Geometry check sheet. Reference: the model listing, model coordinates, mm. A direction names the side the tool comes from. Give positions to 0.01 mm unless a question says otherwise; leave off trailing zeros. Write each loop counter-clockwise with the first axis right and the second up, starting at its lowest first coordinate (ties: lowest second). Pieces come first, ordered by that corner, then holes.
(1) Cross-section at C-C (y = -12). Record the boundary of the cut face in (x, z) (3 decimals).
(2) Depth check by flat-ended pin: P1, Ø0.5, axis at y = -8, z = 4, coming from the -X side; P2, Ø1, axis at x = 12, y = -24, coming from the +Z side. Enter the tip coordinate at first touch or a pass-through.
(3) Cross-section at A-A (y = -6.75). Record the boundary of the cut face in (x, z).
(4) Cross-section at D-D (x = 19.75). Record the boundary of the cut face in (y, z).
(5) Tool access check on faces 3 (the flat face through (3, -5, 4)), 4 (the flat face through (11.875, -27, 1)), 5 (the flat face through (14, -9.4, 1)). Record the directions out of +Z, -Z, +X, -X, +Y, -Y that give a thin tool (end or side, any length) a straight path to the whole face; none if there is none.
(6) Cross-section at B-B (x = 13). Count the separate pieces of the cut face and the enclosed holes in it, and give its area (3 significant figures).
(7) Thickness scan on line 1 along Y through (x, z) = (12.25, 1.4); line 2 along Y through (x, z) = (16.25, 3.15); line 3 along X through (y, z) = (-14.75, 3). Record the ranges inside material, lowest first.
(8) Mould release check, pull along X, two halves, no side actions. Record for faces 1 (the flat face through (3, -8, 4)), 2 (the flat face through (22, -14, 2)): +X half, -X half, draft (parallel to the pull), parting line (faces both ways), or undercut.
Autodesk Inventor part; units mm, degrees
ref_plane "YZ Plane" through (0, 0, 0) normal (1, 0, 0) x (0, 1, 0)
ref_plane "XZ Plane" through (0, 0, 0) normal (0, 1, 0) x (-1, 0, 0)
ref_plane "XY Plane" through (0, 0, 0) normal (0, 0, 1) x (1, 0, 0)
sketch "Sketch1" plane through (0, 0, 0) normal (0, 0, 1) x (1, 0, 0)
  line L0 (0, 0) -> (22, 0)
  line L1 (22, 0) -> (22, -29)
  line L2 (22, -29) -> (0, -29)
  line L3 (0, -29) -> (0, 0)
  line L4 (3, -5.35) -> (19, -5.35)
  line L5 (19, -5.35) -> (19, -7.65)
  line L6 (19, -7.65) -> (3, -7.65)
  line L7 (3, -7.65) -> (3, -5.35)
  line L8 (3, -13.35) -> (19, -13.35)
  line L9 (19, -13.35) -> (19, -15.65)
  line L10 (19, -15.65) -> (3, -15.65)
  line L11 (3, -15.65) -> (3, -13.35)
  line L12 (3, -21.35) -> (19, -21.35)
  line L13 (19, -21.35) -> (19, -23.65)
  line L14 (19, -23.65) -> (3, -23.65)
  line L15 (3, -23.65) -> (3, -21.35)
  line L16 (19, -5.35) -> (19, -13.35) construction
  line L17 (19, -13.35) -> (19, -21.35) construction
  line L18 (22, -14.5) -> (0, -14.5) construction
  line L19 (11, 0) -> (11, -29) construction
  point P0 (19, -14.5)
  point P1 (11, -5.35)
  dimension "d0" = 22
  dimension "d1" = 29
  dimension "d2" = 2.3
  dimension "d3" = 8
  dimension "d4" = 16
extrude "Body with light pipe slots" add sketch "Sketch1" along normal blind 4.5
sketch "Sketch2" plane through (0, 0, 4.5) normal (0, 0, 1) x (1, 0, 0)
  line L0 (0, -29) -> (22, -29) construction
  line L1 (22, -29) -> (22, 0) construction
  line L2 (22, 0) -> (0, 0) construction
  line L3 (0, 0) -> (0, -29) construction
  line L4 (3, -21.35) -> (19, -21.35) construction
  line L5 (19, -21.35) -> (19, -23.65) construction
  line L6 (19, -23.65) -> (3, -23.65) construction
  line L7 (3, -23.65) -> (3, -21.35) construction
  line L8 (3, -13.35) -> (19, -13.35) construction
  line L9 (19, -13.35) -> (19, -15.65) construction
  line L10 (19, -15.65) -> (3, -15.65) construction
  line L11 (3, -15.65) -> (3, -13.35) construction
  line L12 (3, -5.35) -> (19, -5.35) construction
  line L13 (19, -5.35) -> (19, -7.65) construction
  line L14 (19, -7.65) -> (3, -7.65) construction
  line L15 (3, -7.65) -> (3, -5.35) construction
  line L16 (1, -5.35) -> (21, -5.35)
  line L17 (21, -5.35) -> (21, -7.65)
  line L18 (21, -7.65) -> (1, -7.65)
  line L19 (1, -7.65) -> (1, -5.35)
  line L20 (1, -13.35) -> (21, -13.35)
  line L21 (21, -13.35) -> (21, -15.65)
  line L22 (21, -15.65) -> (1, -15.65)
  line L23 (1, -15.65) -> (1, -13.35)
  line L24 (1, -21.35) -> (21, -21.35)
  line L25 (21, -21.35) -> (21, -23.65)
  line L26 (21, -23.65) -> (1, -23.65)
  line L27 (1, -23.65) -> (1, -21.35)
  dimension "d7" = 2
  dimension "d8" = 2
extrude "Light pipe wing cuts" cut sketch "Sketch2" against normal blind 4
sketch "Sketch3" plane through (0, 0, 4.5) normal (0, 0, 1) x (1, 0, 0)
  line L0 (1, -21.35) -> (21, -21.35) construction
  line L1 (21, -21.35) -> (21, -23.65) construction
  line L2 (21, -23.65) -> (1, -23.65) construction
  line L3 (1, -23.65) -> (1, -21.35) construction
  line L4 (1, -13.35) -> (21, -13.35) construction
  line L5 (21, -13.35) -> (21, -15.65) construction
  line L6 (21, -15.65) -> (1, -15.65) construction
  line L7 (1, -15.65) -> (1, -13.35) construction
  line L8 (1, -5.35) -> (21, -5.35) construction
  line L9 (21, -5.35) -> (21, -7.65) construction
  line L10 (21, -7.65) -> (1, -7.65) construction
  line L11 (1, -7.65) -> (1, -5.35) construction
  line L12 (0, -29) -> (22, -29) construction
  line L13 (22, -29) -> (22, 0) construction
  line L14 (22, 0) -> (0, 0) construction
  line L15 (0, 0) -> (0, -29) construction
  line L16 (3, -5.35) -> (3, -7.65) construction
  line L17 (19, -7.65) -> (19, -5.35) construction
  line L18 (19, -15.65) -> (19, -13.35) construction
  line L19 (19, -23.65) -> (19, -21.35) construction
  line L20 (3, -21.35) -> (3, -23.65) construction
  line L21 (3, -13.35) -> (3, -15.65) construction
  line L22 (3, -4.35) -> (19, -4.35)
  line L23 (19, -4.35) -> (19, -8.65)
  line L24 (19, -8.65) -> (3, -8.65)
  line L25 (3, -8.65) -> (3, -4.35)
  line L26 (3, -12.35) -> (19, -12.35)
  line L27 (19, -12.35) -> (19, -16.65)
  line L28 (19, -16.65) -> (3, -16.65)
  line L29 (3, -16.65) -> (3, -12.35)
  line L30 (3, -20.2545) -> (19, -20.2545)
  line L31 (19, -20.2545) -> (19, -24.5545)
  line L32 (19, -24.5545) -> (3, -24.5545)
  line L33 (3, -24.5545) -> (3, -20.2545)
  dimension "d11" = 1
  dimension "d12" = 1
  dimension "d13" = 1.0956
  dimension "d14" = 1
extrude "SMD clearance cuts" cut sketch "Sketch3" against normal blind 1
sketch "Sketch4" plane through (0, 0, 0) normal (0, 0, -1) x (-1, 0, 0)
  line L0 (-22, 0) -> (0, 0) construction
  line L1 (-11, 0) -> (-11, -29) construction
  line L2 (0, -29) -> (-22, -29) construction
  line L3 (-11.875, 0) -> (-10.125, 0)
  line L4 (-10.125, -29) -> (-11.875, -29)
  line L5 (-3, -5.35) -> (-19, -5.35)
  line L6 (-19, -23.65) -> (-3, -23.65)
  line L7 (-6.75, -23.65) -> (-6.75, -25.4)
  line L8 (-15.25, -25.4) -> (-15.25, -23.65)
  line L9 (-19, -15.65) -> (-3, -15.65)
  line L10 (-6.75, -15.65) -> (-6.75, -17.4)
  line L11 (-15.25, -17.4) -> (-15.25, -15.65)
  line L12 (-3, -7.65) -> (-19, -7.65)
  line L13 (-6.75, -7.65) -> (-6.75, -9.4)
  line L14 (-15.25, -9.4) -> (-15.25, -7.65)
  line L15 (-11.875, -7.65) -> (-11.875, 0)
  line L16 (-10.125, 0) -> (-10.125, -7.65)
  line L17 (-6.75, -9.4) -> (-10.125, -9.4)
  line L18 (-11.875, -9.4) -> (-15.25, -9.4)
  line L19 (-11.875, -15.65) -> (-11.875, -9.4)
  line L20 (-10.125, -9.4) -> (-10.125, -15.65)
  line L21 (-15.25, -15.65) -> (-11.875, -15.65)
  line L22 (-10.125, -15.65) -> (-6.75, -15.65)
  line L23 (-6.75, -17.4) -> (-10.125, -17.4)
  line L24 (-11.875, -17.4) -> (-15.25, -17.4)
  line L25 (-15.25, -23.65) -> (-11.875, -23.65)
  line L26 (-10.125, -23.65) -> (-6.75, -23.65)
  line L27 (-6.75, -25.4) -> (-10.125, -25.4)
  line L28 (-11.875, -25.4) -> (-15.25, -25.4)
  line L29 (-11.875, -29) -> (-11.875, -25.4)
  line L30 (-11.875, -23.65) -> (-11.875, -17.4)
  line L31 (-10.125, -17.4) -> (-10.125, -23.65)
  line L32 (-10.125, -25.4) -> (-10.125, -29)
  line L33 (-15.25, -7.65) -> (-11.875, -7.65)
  line L34 (-10.125, -7.65) -> (-6.75, -7.65)
  point P0 (-10.125, -7.65)
  dimension "d18" = 1.75
  dimension "d20" = 1.75
  dimension "d21" = 8.5
  dimension "d22" = 4.25
extrude "Case interior molding cuts" cut sketch "Sketch4" against normal blind 3
equation "\"d8\" = d7"
equation "\"d12\" = d11"
equation "\"d14\" = d11"
equation "\"d22\" = 0.5 * d21"
properties part number "Lightpipe shield"
Reply:
1. outline: (0, 0) - (10.125, 0) - (10.125, 3) - (11.875, 3) - (11.875, 0) - (22, 0) - (22, 4.5) - (0, 4.5) - close
2. P1: stops at x = 0
2. P2: stops at z = 3.5
3. outline: (0, 0) - (3, 0) - (3, 0.5) - (1, 0.5) - (1, 4.5) - (0, 4.5) - close; (19, 0) - (22, 0) - (22, 4.5) - (21, 4.5) - (21, 0.5) - (19, 0.5) - close
4. outline: (-29, 0) - (0, 0) - (0, 4.5) - (-5.35, 4.5) - (-5.35, 0.5) - (-7.65, 0.5) - (-7.65, 4.5) - (-13.35, 4.5) - (-13.35, 0.5) - (-15.65, 0.5) - (-15.65, 4.5) - (-21.35, 4.5) - (-21.35, 0.5) - (-23.65, 0.5) - (-23.65, 4.5) - (-29, 4.5) - close
5. face 3: +Z
5. face 4: -Z, +Y, -Y
5. face 5: -Z
6. separate pieces: 4
6. enclosed holes: 0
6. area: 77.7 mm2
7. line 1: y = -29 to -25.4, -21.35 to -17.4, -13.35 to -9.4, -5.35 to 0
7. line 2: y = -29 to -23.65, -21.35 to -15.65, -13.35 to -7.65, -5.35 to 0
7. line 3: x = 0 to 1, 21 to 22
8. face 1: undercut
8. face 2: +X half
